Read the model definition and answer for the solid it produces. Units are mm, in the model's axes. A direction names the side the tool comes from. Coordinates: 2 decimals unless noted, no trailing zeros. Loops run counter-clockwise (first coordinate to the right, second up) from the corner with the lowest first, then second, coordinate; pieces in that order, holes last.
Q1. Flat-ended cylindrical pins translate along their axes: P1, Ø8, axis at x = 29.5, z = 9, coming from the -Y side; P2, Ø5, axis at y = 5, z = 20, coming from the -X side; P3, Ø3.5, axis at x = -25.5, y = 3.5, coming from the +Z side. Find the tip coordinate at first contact, or state that the pin passes through.
Q2. Section A-A (y = 55) is taken. Give the vertices of the cut face in (x, z).
Q3. Straight lines are drawn through the part: line 1 (Y direction, x = 8, z = 12.75); line 2 (Y direction, x = 22, z = 22); line 3 (Z direction, x = -17.5, y = -7). For each, find the intervals that lie inside material, in ascending order.
Q4. Which of the six approach directions +Z, -Z, +X, -X, +Y, -Y give full straight-line access (tool end or side, diameter ignored) to faces 5 (the face through (27.5, 3.6, 13.9)), 6 (the face through (18.34, 52.22, 1.97)), 7 (the face through (22, 49, 4)), 8 (the face through (30.134, 29.32, 1.972)), 9 (the face through (0, -24, 13.5))?
Q5. Section B-B (z = 25.5) is taken. Give the vertices of the cut face in (x, y), then the cut area to 3 significant figures.
Q6. Section D-D (y = -7) is taken. Give the vertices of the cut face in (x, z), then the cut area to 3 significant figures.
Q7. Section C-C (z = 19) is taken. Give the vertices of the cut face in (x, y).
Q8. The mould has two halves that part along X. Classify faces 1 (the face through (3.583, 38.279, 13.86)), 2 (the face through (24.306, 19.235, 4.285)), 3 (the face through (-12.878, 42.457, 4.285)), 4 (the face through (34, 26, 4)): pulls with the +X half, pulls with the -X half, needs draft (parallel to the pull), parting line crosses it, or undercut.
from build123d import *

# Parameters (mm, degrees)
BASE_SHELL_DEPTH         = 30
COQUE1_T                 = -2
COQUE1_THICKNESS_2_DEPTH = 2
ESQUISSE4_R              = 1.5
BOSS_EXTRU_2_DEPTH       = 24
ESQUISSE6_R              = 2.5
BOSS_EXTRU_3_DEPTH       = 4
CONG_2_R                 = 1
ENL_V_MAT_EXTRU_1_DEPTH  = 2
CONG_3_R                 = 0.3


with BuildPart() as part:
    # Esquisse2 → Base shell (new body)
    with BuildSketch(Plane.XY):
        with BuildLine():
            Line((-26.917573139, 13.245537222), (-4.48626219, 58.830434456))
            ThreePointArc((-4.48626219, 58.830434456), (0, 61.622844919), (4.48626219, 58.830434456))
            Line((4.48626219, 58.830434456), (26.917573139, 13.245537222))
            ThreePointArc((26.917573139, 13.245537222), (28.868799962, -8.160415969), (16, -25.377155081))
            Line((16, -25.377155081), (-16, -25.377155081))
            ThreePointArc((-16, -25.377155081), (-28.868799962, -8.160415969), (-26.917573139, 13.245537222))
        make_face()
    extrude(amount=BASE_SHELL_DEPTH)

    # Coque1
    coque1_openings = [part.faces().sort_by_distance(p)[0] for p in [
        (0, 9.805982993, 30),
    ]]
    offset(amount=COQUE1_T, openings=coque1_openings, kind=Kind.INTERSECTION)

    # Coque1 thickness 2 face (on inner face of the shell) → Coque1 thickness 2 (add)
    with BuildSketch(Plane(origin=(0, 9.437987549, 2), x_dir=(-1, 0, 0), z_dir=(0, 0, -1))):
        with BuildLine():
            Line((2.691757314, 48.509411092), (25.123068263, 2.924513858))
            ThreePointArc((25.123068263, 2.924513858), (27.020174162, -16.780343321), (15.411314685, -32.81514263))
            Line((15.411314685, -32.81514263), (-15.411314685, -32.81514263))
            ThreePointArc((-15.411314685, -32.81514263), (-27.020174162, -16.780343321), (-25.123068263, 2.924513858))
            Line((-25.123068263, 2.924513858), (-2.691757314, 48.509411092))
            ThreePointArc((-2.691757314, 48.509411092), (0, 50.18485737), (2.691757314, 48.509411092))
        make_face()
    extrude(amount=-COQUE1_THICKNESS_2_DEPTH)

    # Esquisse4 → Boss.-Extru.2 (add)
    # profile 1 of 4: a face of its own
    with BuildSketch(Plane.XY):
        with BuildLine():
            Line((-8.787069617, 45.560508478), (-12.392350614, 38.233858506))
            ThreePointArc((-12.392350614, 38.233858506), (-3.51373781, 38.415255382), (-8.787069617, 45.560508478))
        make_face()
        with Locations((-8, 40.622844919)):
            Circle(ESQUISSE4_R, mode=Mode.SUBTRACT)
    # profile 2 of 4: a face of its own
    with BuildSketch(Plane.XY):
        with BuildLine():
            Line((8.787069617, 45.560508478), (12.392350614, 38.233858506))
            ThreePointArc((12.392350614, 38.233858506), (3.51373781, 38.415255382), (8.787069617, 45.560508478))
        make_face()
        with Locations(Location((8, 40.622844919, 0), (0, 0, 180))):
            Circle(ESQUISSE4_R, mode=Mode.SUBTRACT)
    # profile 3 of 4: a face of its own
    with BuildSketch(Plane.XY):
        with BuildLine():
            ThreePointArc((-27.983297548, -0.966984145), (-21.047843649, 2.932810516), (-26.653016398, 8.580018467))
            ThreePointArc((-26.653016398, 8.580018467), (-27.732075565, 3.864192656), (-27.983297548, -0.966984145))
        make_face()
        with Locations((-26, 3.622844919)):
            Circle(ESQUISSE4_R, mode=Mode.SUBTRACT)
    # profile 4 of 4: a face of its own
    with BuildSketch(Plane.XY):
        with BuildLine():
            ThreePointArc((27.983297548, -0.966984145), (21.047843649, 2.932810516), (26.653016398, 8.580018467))
            ThreePointArc((26.653016398, 8.580018467), (27.732075565, 3.864192656), (27.983297548, -0.966984145))
        make_face()
        with Locations(Location((26, 3.622844919, 0), (0, 0, 180))):
            Circle(ESQUISSE4_R, mode=Mode.SUBTRACT)
    extrude(amount=BOSS_EXTRU_2_DEPTH)

    # Esquisse6 → Boss.-Extru.3 (add)
    # profile 1 of 2: a face of its own
    with BuildSketch(Plane.XY):
        with BuildLine():
            Line((0, 36.165725179), (-24.951408489, 58.009624237))
            ThreePointArc((-24.951408489, 58.009624237), (-30.595831001, 57.634798275), (-30.221005039, 51.990375763))
            Line((-30.221005039, 51.990375763), (0, 25.533168595))
            Line((0, 25.533168595), (0, 36.165725179))
        make_face()
        with Locations((-27.586206764, 55)):
            Circle(ESQUISSE6_R, mode=Mode.SUBTRACT)
    # profile 2 of 2: a face of its own
    with BuildSketch(Plane.XY):
        with BuildLine():
            Line((0, 2.938985855), (-37.122207588, 35.437902929))
            ThreePointArc((-37.122207588, 35.437902929), (-42.7666301, 35.063076966), (-42.391804138, 29.418654454))
            Line((-42.391804138, 29.418654454), (0, -7.693570729))
            Line((0, -7.693570729), (0, 2.938985855))
        make_face()
        with Locations((-39.757005863, 32.428278691)):
            Circle(ESQUISSE6_R, mode=Mode.SUBTRACT)
    boss_extru_3 = extrude(amount=BOSS_EXTRU_3_DEPTH)

    # Symétrie1: Boss.-Extru.3 across plane
    add(boss_extru_3.mirror(Plane(origin=(0, 0, 0), x_dir=(0, 0, 1), z_dir=(1, 0, 0))))

    # Congé2
    cong_2_edges = [part.edges().sort_by_distance(p)[0] for p in [
        (-14.587086989, 38.303544098, 2),
        (-10.930343207, 45.734776713, 2),
        (-24.186039417, 18.796558485, 4),
        (-22.357667526, 22.512174792, 2),
        (-26.014411308, 15.080942177, 2),
        (12.758715098, 42.019160406, 4),
        (14.587086989, 38.303544098, 2),
        (10.930343207, 45.734776713, 2),
        (24.186039417, 18.796558485, 4),
        (22.357667526, 22.512174792, 2),
        (26.014411308, 15.080942177, 2),
        (-12.758715098, 42.019160406, 4),
    ]]
    fillet(cong_2_edges, radius=CONG_2_R)

    # Esquisse8 → Enlèv. mat.-Extru.1 (cut)
    with BuildSketch(Plane.XZ.offset(25.377155081)):
        Polygon((2.5, 12), (-2.5, 12), (-4.5, 12.75), (-4.5, 13.5), (4.5, 13.5), (4.5, 12.75), align=None)
    extrude(amount=-ENL_V_MAT_EXTRU_1_DEPTH, mode=Mode.SUBTRACT)

    # Congé3
    cong_3_edges = [part.edges().sort_by_distance(p)[0] for p in [
        (2.5, -24.377155081, 12),
        (4.5, -24.377155081, 12.75),
        (4.5, -24.377155081, 13.5),
        (-4.5, -24.377155081, 13.5),
        (-4.5, -24.377155081, 12.75),
        (-2.5, -24.377155081, 12),
    ]]
    fillet(cong_3_edges, radius=CONG_3_R)


solid = part.part
Numbers:
1. P1: stops at y = -15.8
1. P2: stops at x = -29.9
1. P3: stops at z = 24
2. outline: (-31.59, 0) - (-30.09, 0) - (-30.09, 4) - (-31.59, 4) - close; (-25.09, 0) - (-21.51, 0) - (-21.51, 4) - (-25.09, 4) - close; (-6.37, 0) - (6.37, 0) - (6.37, 30) - (4.14, 30) - (4.14, 4) - (-4.14, 4) - (-4.14, 30) - (-6.37, 30) - close; (21.51, 0) - (25.09, 0) - (25.09, 4) - (21.51, 4) - close; (30.09, 0) - (31.59, 0) - (31.59, 4) - (30.09, 4) - close
3. line 1: y = -25.38 to -23.38, 35.62 to 39.12, 42.12 to 45.62, 47.16 to 51.69
3. line 2: y = -20.4 to -17.32, 0.62 to 6.62, 18.71 to 23.24
3. line 3: z = 0 to 4
4. face 5: +Z
4. face 6: +Z, -Z, +Y
4. face 7: +Z, +X, +Y
4. face 8: +Z, -Z
4. face 9: -Y
5. outline: (-26.92, 13.25) arc R30 ccw to (-16, -25.38) - (16, -25.38) arc R30 ccw to (26.92, 13.25) - (4.49, 58.83) arc R5 ccw to (-4.49, 58.83) - close; hole (-25.12, 12.36) arc R28 ccw to (-15.41, -23.38) - (15.41, -23.38) arc R28 ccw to (25.12, 12.36) - (2.69, 57.95) arc R3 ccw to (-2.69, 57.95) - close
5. area: 453 mm2
6. outline: (-29.17, 0) - (29.17, 0) - (29.17, 30) - (27.11, 30) - (27.11, 4) - (-27.11, 4) - (-27.11, 30) - (-29.17, 30) - close
6. area: 341 mm2
7. outline: (-26.92, 13.25) arc R30 ccw to (-16, -25.38) - (16, -25.38) arc R30 ccw to (26.92, 13.25) - (4.49, 58.83) arc R5 ccw to (-4.49, 58.83) - close; hole (-27.98, -0.97) arc R28 ccw to (-15.41, -23.38) - (15.41, -23.38) arc R28 ccw to (27.98, -0.97) arc R5 cw (long way) to (26.65, 8.58) arc R28 ccw to (25.12, 12.36) - (12.39, 38.23) arc R5 cw (long way) to (8.79, 45.56) - (2.69, 57.95) arc R3 ccw to (-2.69, 57.95) - (-8.79, 45.56) arc R5 cw (long way) to (-12.39, 38.23) - (-25.12, 12.36) arc R28 ccw to (-26.65, 8.58) arc R5 cw (long way) to start; hole circle Ø3 at (-26, 3.62); hole circle Ø3 at (-8, 40.62); hole circle Ø3 at (8, 40.62); hole circle Ø3 at (26, 3.62)
8. face 1: undercut
8. face 2: pulls with the +X half
8. face 3: pulls with the -X half
8. face 4: needs draft
